Input: dimensioned drawing with shaded views. Units: mm. Origin: part minimum x, y, z. Round coordinates to 2 decimals unless told otherwise and drop trailing zeros. Loops run counter-clockwise (first coordinate to the right, second up) from the corner with the lowest first, then second, coordinate; pieces in that order, holes last.
1) Draft query along X for the marked faces 1, 2, 3 and 4. Return one class per face: pulls with the +X half, pulls with the -X half, needs draft (parallel to the pull), parting line crosses it, or undercut.
2) Section D-D, the plane x = 666. Return loops of the section in (y, z) (1 decimal).
3) Section A-A, the plane z = 605. Return loops of the section in (x, y).
4) First-contact query: pin 1 (4 mm diameter, centred on y = 281, z = 440, fed in from -X); pin 2 (5 mm diameter, centred on x = 232, y = 524.5, fed in from -Z). Flat tips, straight axial feed; report the tip coordinate or a pass-through.
5) Section B-B, the plane z = 819.5. Return loops of the section in (x, y).
6) Ray query, line 1 along X through (y, z) = (238, 746); line 2 along Z through (x, y) = (58.5, 206.5); line 3 along Y through (x, z) = (398, 765.5). Return the intervals inside material, ascending.
7) Section C-C, the plane y = 88.5. Return loops of the section in (x, z), and give its area (3 significant figures).
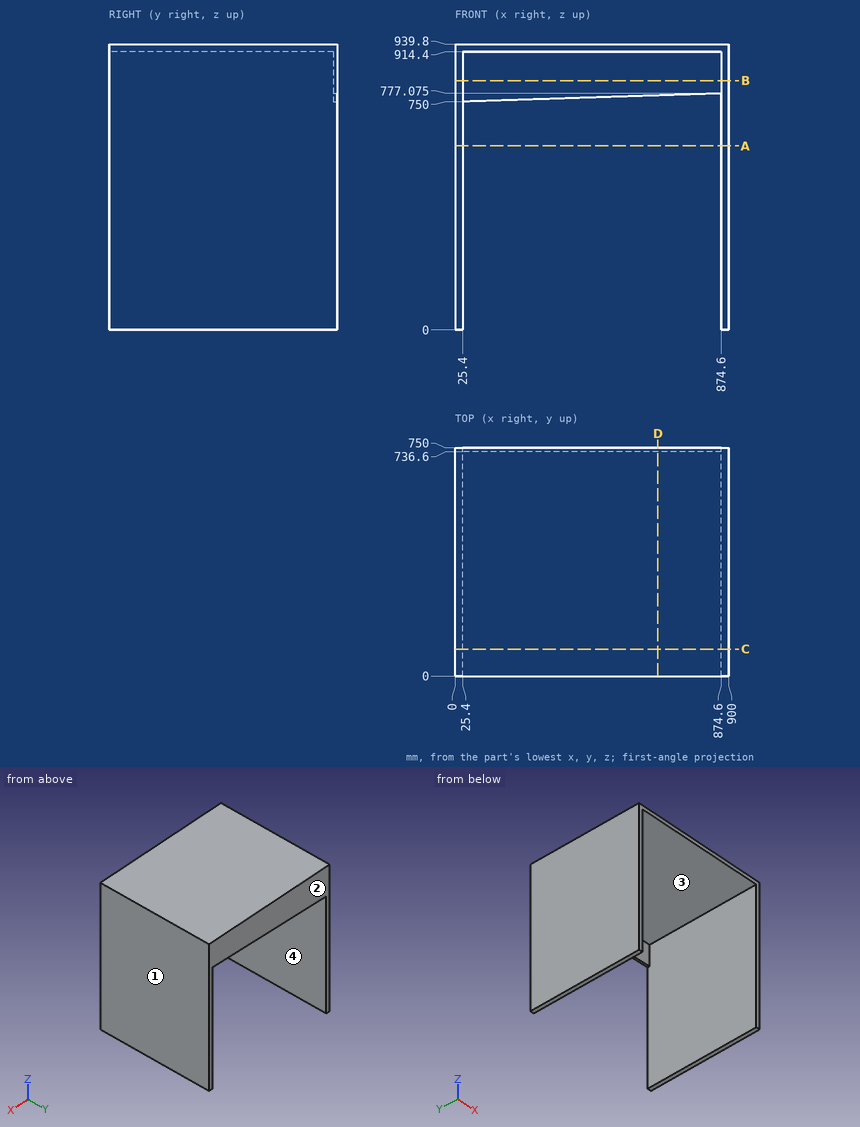
Final values:
1. face 1: pulls with the +X half
1. face 2: needs draft
1. face 3: undercut
1. face 4: undercut
2. outline: (0, 914.4) - (736.6, 914.4) - (736.6, 770.4) - (750, 770.4) - (750, 939.8) - (0, 939.8) - close
3. outline: (0, 0) - (25.4, 0) - (25.4, 750) - (0, 750) - close; (874.6, 0) - (900, 0) - (900, 750) - (874.6, 750) - close
4. pin 1: stops at x = 0
4. pin 2: stops at z = 914.4
5. outline: (0, 0) - (25.4, 0) - (25.4, 736.6) - (874.6, 736.6) - (874.6, 0) - (900, 0) - (900, 750) - (0, 750) - close
6. line 1: x = 0 to 25.4, 874.6 to 900
6. line 2: z = 914.4 to 939.8
6. line 3: y = 736.6 to 750
7. outline: (0, 0) - (25.4, 0) - (25.4, 914.4) - (874.6, 914.4) - (874.6, 0) - (900, 0) - (900, 939.8) - (0, 939.8) - close
7. area: 69,300 mm2
